Read the model definition and answer for the solid it produces. Units are mm, in the model's axes. A direction names the side the tool comes from. Coordinates: 2 decimals unless noted, no trailing zeros. Loops run counter-clockwise (first coordinate to the right, second up) from the corner with the lowest first, then second, coordinate; pieces in that order, holes last.
Q1. Section C-C (x = 16.25) is taken. Give the vertices of the cut face in (y, z).
Q2. Which of the six approach directions +Z, -Z, +X, -X, +Y, -Y give full straight-line access (tool end or side, diameter ignored) to faces 4 (the face through (0.904, 5.325, 5.309)), 5 (the face through (0.903, -5.135, -4.029)), 6 (the face through (0.903, -2.167, 5.285)), 7 (the face through (0.903, -4.05, -5.156)), 8 (the face through (23.261, -3.827, -0.502))?
Q3. Flat-ended cylindrical pins translate along their axes: P1, Ø8, axis at x = 19, z = 6, coming from the -Y side; P2, Ø0.5, axis at x = 1, y = -7, coming from the -Z side; P3, Ø3, axis at x = 21.5, z = 1.5, coming from the -Y side; P4, Ø1.5, axis at x = 21.5, y = -5, coming from the -Z side. Find the tip coordinate at first contact, or state that the pin passes through.
Q4. The mould has two halves that part along Y. Classify faces 1 (the face through (0.9, -2.2, -5.27)), 2 (the face through (1, 7, 0.782)), 3 (the face through (0.904, 5.309, -5.325)): pulls with the +Y half, pulls with the -Y half, needs draft (parallel to the pull), parting line crosses it, or undercut.
Q5. Straight lines are drawn through the part: line 1 (X direction, y = -2.75, z = -6.25); line 2 (Y direction, x = 11.75, z = -0.5); line 3 (X direction, y = 4.75, z = -1.75). For each, find the intervals that lie inside material, in ascending order.
from build123d import *

# Parameters (mm, degrees)
RIBCUT_START     = -1.832
RIBCUT_DEPTH     = 1.832
RIBCUTSPAT_COUNT = 8
RIBCUTSPAT_ANGLE = 315


with BuildPart() as part:
    # BodySke → BaseBody (revolve)
    with BuildSketch(Plane.XY, mode=Mode.PRIVATE) as basebody_sk:
        with BuildLine():
            Line((-2.29, 7.392), (-2.29, 0))
            Line((-2.29, 0), (25, 0))
            Line((25, 0), (25, 3.86))
            Line((25, 3.86), (21.57, 3.86))
            Line((21.57, 3.86), (21.258, 4.172))
            Line((21.258, 4.172), (17.2, 5))
            Line((17.2, 5), (1.832, 5))
            Line((1.832, 5), (1.832, 7.181591015))
            Line((1.832, 7.181591015), (0.00254, 7.84746))
            Line((0.00254, 7.84746), (0, 7.84746))
            Line((0, 7.84746), (0, 7.85))
            Line((0, 7.85), (-1.832, 7.85))
            ThreePointArc((-1.832, 7.85), (-2.155854906, 7.715854906), (-2.29, 7.392))
        make_face()
    revolve(basebody_sk.sketch.rotate(Axis((0, 0, 0), (1, 0, 0)), 90), axis=Axis((0, 0, 0), (1, 0, 0)))

    # RibCutSke → RibCut (cut)
    with BuildSketch(Plane(origin=(1.832, 1.794401132, -0.090952894), x_dir=(0, 0, -1), z_dir=(1, 0, 0)).offset(RIBCUT_START)):
        with BuildLine():
            Line((0.691219431, 3.864296837), (0.691219431, 6.016533924))
            ThreePointArc((0.691219431, 6.016533924), (2.91311205, 5.458053198), (4.879132896, 4.281843369))
            Line((4.879132896, 4.281843369), (3.357271457, 2.759981929))
            ThreePointArc((3.357271457, 2.759981929), (2.095126213, 3.483260697), (0.691219431, 3.864296837))
        make_face()
    ribcut = extrude(amount=RIBCUT_DEPTH, mode=Mode.SUBTRACT)

    # RibCutsPat: RibCut ×8 about axis
    ribcutspat_axis = Axis((0, 0, 0), (1, 0, 0))
    for i in range(1, RIBCUTSPAT_COUNT):
        add(ribcut.rotate(ribcutspat_axis, i * RIBCUTSPAT_ANGLE / (RIBCUTSPAT_COUNT - 1)), mode=Mode.SUBTRACT)


solid = part.part
Numbers:
1. outline: circle Ø10 at (0, 0)
2. face 4: +Z, +X, +Y
2. face 5: +X, -Y
2. face 6: +Z, +X
2. face 7: -Z, +X
2. face 8: +X
3. P1: stops at y = -4.38
3. P2: stops at z = -0.78
3. P3: stops at y = -4.33
3. P4: passes through
4. face 1: undercut
4. face 2: needs draft
4. face 3: pulls with the +Y half
5. line 1: x = -2.29 to 0
5. line 2: y = -4.97 to 4.97
5. line 3: x = -2.29 to 1.83
